Build history of the part. All positions in model axes, mm. A direction names the side the tool comes from. Round coordinates to 2 decimals unless told otherwise and drop trailing zeros. Loops run counter-clockwise (first coordinate to the right, second up) from the corner with the lowest first, then second, coordinate; pieces in that order, holes last. Notation, with made-up numbers: (-29, 39) -> (-16, 39) arc R17 ccw to (-16, 45) -> close; hole circle Ø6 at (84, 89.25). An arc over 180 degrees is marked (long way). Put each result on its own line as item: value. Start each with the question number.
```python
from build123d import *

# Parameters (mm, degrees)
SKETCH_1_R      = 18.25
EXTRUDE_1_DEPTH = 20
FILLET_1_R      = 2
SKETCH_2_R      = 10
EXTRUDE_2_DEPTH = 1.6
SKETCH_3_R      = 3
EXTRUDE_3_DEPTH = 19
FILLET_2_R      = 0.5


with BuildPart() as part:
    # 草图1 → 凸台-拉伸1 (new body)
    with BuildSketch(Plane(origin=(0, 0, 0), x_dir=(1, 0, 0), z_dir=(0, 1, 0))):
        with Locations(Location((0, 0, 0), (0, 0, 270))):
            Circle(SKETCH_1_R)
    extrude(amount=EXTRUDE_1_DEPTH)

    # 圆角1
    fillet_1_edges = [part.edges().sort_by_distance(p)[0] for p in [
        (0, 0, -18.25),
        (0, 20, -18.25),
    ]]
    fillet(fillet_1_edges, radius=FILLET_1_R)

    # 草图2 → 凸台-拉伸2 (add)
    with BuildSketch(Plane(origin=(0, 0, 0), x_dir=(1, 0, 0), z_dir=(0, 1, 0))):
        with Locations(Location((0, 0, 0), (0, 0, 270))):
            Circle(SKETCH_2_R)
    extrude(amount=-EXTRUDE_2_DEPTH)

    # 草图3 → 凸台-拉伸3 (add)
    with BuildSketch(Plane(origin=(0, 0, 0), x_dir=(1, 0, 0), z_dir=(0, 1, 0))):
        with Locations(Location((0, 0, 0), (0, 0, 270))):
            Circle(SKETCH_3_R)
    extrude(amount=-EXTRUDE_3_DEPTH)

    # 圆角2
    fillet_2_edges = [part.edges().sort_by_distance(p)[0] for p in [
        (0, -19, -3),
    ]]
    fillet(fillet_2_edges, radius=FILLET_2_R)


solid = part.part
```
Item 1: 3-axis set-ups, long thin cutter, end or side, ignore diameter. For faces 1 (the face through (-17.816, 9.888, -3.956)), 2 (the face through (0.9, -9.93, 2.86)): which of +Z, -Z, +X, -X, +Y, -Y reach the whole face in a straight line?
Item 2: Cut at B-B on x = 0. Write the cut outline in (y, z), then the cut area to 3 significant figures.
Item 3: Drop flat-ended pins along their axis: pin 1 (3 mm diameter, centred on x = -11, y = -4.5, fed in from +Z); pin 2 (6 mm diameter, centred on y = 2.5, z = 7.5, fed in from -X); pin 3 (6 mm diameter, centred on y = 15.5, z = -13, fed in from +X); pin 4 (10 mm diameter, centred on y = 14, z = -7, fed in from +X). Give the stop position or say it passes through.
Item 4: Cut at A-A on z = 0. Write the cut outline in (x, y), then the cut area to 3 significant figures.
Item 5: Wall check: line 1 (Y direction, x = 6, z = 4); line 2 (Y direction, x = -7, z = -11); line 3 (Z direction, x = 11, y = 14.5). Give the ranges that are in metal, low to high. Write a range as from..to.
Item 6: Cut at C-C on y = 13. Write the cut outline in (x, z).
Ans:
1. face 1: +Y, -Y
1. face 2: -Y
2. outline: (-19, -2.5) arc R0.5 ccw to (-18.5, -3) -> (-1.6, -3) -> (-1.6, -10) -> (0, -10) -> (0, -16.25) arc R2 ccw to (2, -18.25) -> (18, -18.25) arc R2 ccw to (20, -16.25) -> (20, 16.25) arc R2 ccw to (18, 18.25) -> (2, 18.25) arc R2 ccw to (0, 16.25) -> (0, 10) -> (-1.6, 10) -> (-1.6, 3) -> (-18.5, 3) arc R0.5 ccw to (-19, 2.5) -> close
2. area: 863 mm2
3. pin 1: passes through
3. pin 2: stops at x = -17.69
3. pin 3: stops at x = 15.27
3. pin 4: stops at x = 18.14
4. outline: (-18.25, 2) arc R2 ccw to (-16.25, 0) -> (-10, 0) -> (-10, -1.6) -> (-3, -1.6) -> (-3, -18.5) arc R0.5 ccw to (-2.5, -19) -> (2.5, -19) arc R0.5 ccw to (3, -18.5) -> (3, -1.6) -> (10, -1.6) -> (10, 0) -> (16.25, 0) arc R2 ccw to (18.25, 2) -> (18.25, 18) arc R2 ccw to (16.25, 20) -> (-16.25, 20) arc R2 ccw to (-18.25, 18) -> close
4. area: 863 mm2
5. line 1: y = -1.6..20
5. line 2: y = 0..20
5. line 3: z = -14.56..14.56
6. outline: circle Ø36.5 at (0, 0)
